Source: three-view drawing plus pictorial views. Frame: mm from the lowest corner of the part. Give positions to 0.01 mm unless a question says otherwise; leave off trailing zeros. Order: outer loops, then holes, each group sorted by start corner. A loop starts at its lowest first (then second) coordinate and runs counter-clockwise, first axis right, second up.
1) Section B-B, the plane x = 70. Return loops of the section in (y, z), plus the area to 3 significant figures.
2) Section A-A, the plane z = 50. Return loops of the section in (x, y) (1 decimal).
3) First-contact query: P1, Ø4, axis at x = 70, z = 89, coming from the -Y side; P2, Ø2, axis at x = 30, z = 89, coming from the +Y side; P3, Ø6, axis at x = 54, y = 3, coming from the -Z side; P4, Ø2, axis at x = 59, y = 10, coming from the +Z side. Flat tips, straight axial feed; report the tip coordinate or a pass-through.
4) Draft query along Y for the marked faces 1, 2 and 3. Return one class per face: released by +Y, released by -Y, zero draft, split by the parting line, or undercut.
5) Section D-D, the plane x = 54. Return loops of the section in (y, z).
6) Material intervals for line 1 (X direction, y = 15.6, z = 89); line 2 (X direction, y = 16.1, z = 15); line 3 (Y direction, x = 76, z = 84), sorted ascending.
7) Section C-C, the plane z = 15. Return loops of the section in (x, y).
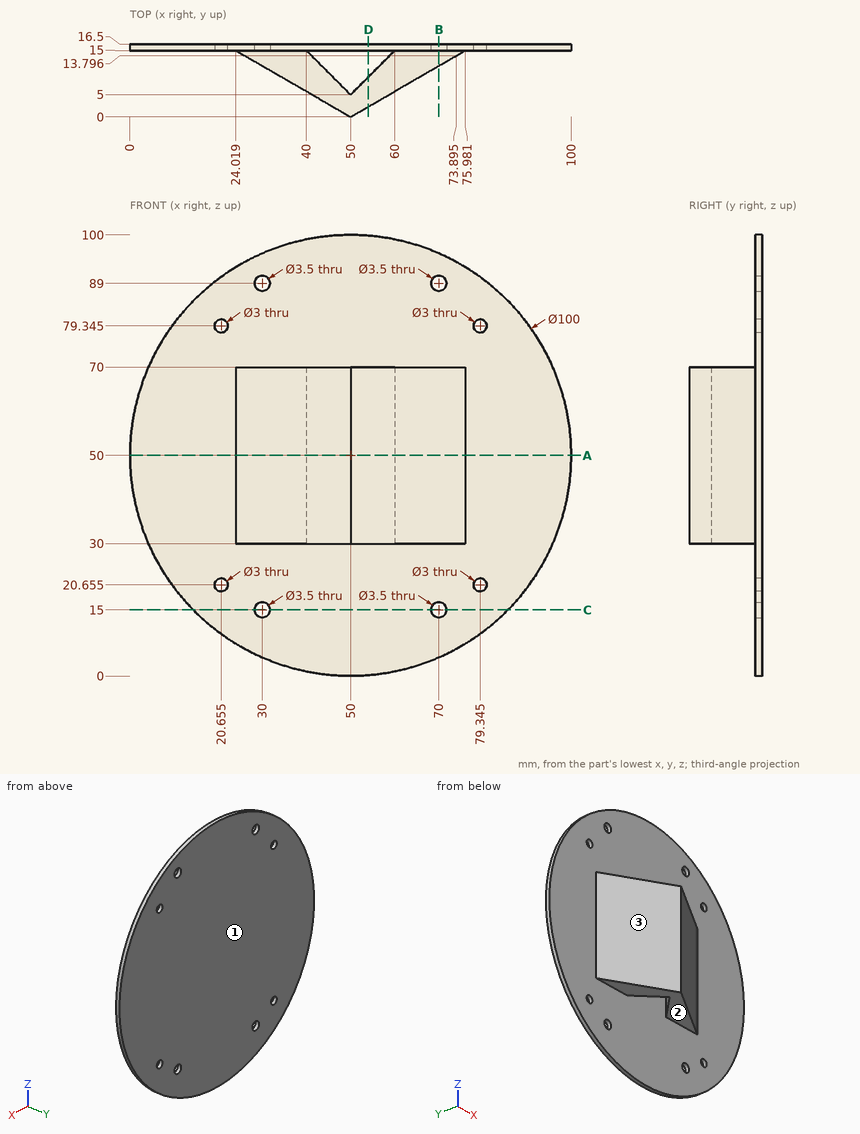
From the geometry:
1. outline: (11.55, 30) - (15, 30) - (15, 16.75) - (16.5, 16.75) - (16.5, 87.25) - (15, 87.25) - (15, 70) - (11.55, 70) - close; (15, 4.17) - (16.5, 4.17) - (16.5, 13.25) - (15, 13.25) - close; (15, 90.75) - (16.5, 90.75) - (16.5, 95.83) - (15, 95.83) - close
1. area: 265 mm2
2. outline: (0, 15) - (24, 15) - (50, 0) - (73.9, 13.8) - (76, 15) - (100, 15) - (100, 16.5) - (0, 16.5) - close; hole (40, 15) - (50, 5) - (60, 15) - close
3. P1: stops at y = 15
3. P2: passes through
3. P3: stops at z = 30
3. P4: stops at z = 70
4. face 1: released by +Y
4. face 2: zero draft
4. face 3: released by -Y
5. outline: (2.31, 30) - (9, 30) - (9, 70) - (2.31, 70) - close; (15, 0.16) - (16.5, 0.16) - (16.5, 99.84) - (15, 99.84) - close
6. line 1: x = 18.71 to 28.25, 31.75 to 68.25, 71.75 to 81.29
6. line 2: x = 14.29 to 28.25, 31.75 to 68.25, 71.75 to 85.71
6. line 3: y = 15 to 16.5
7. outline: (14.29, 15) - (28.25, 15) - (28.25, 16.5) - (14.29, 16.5) - close; (31.75, 15) - (68.25, 15) - (68.25, 16.5) - (31.75, 16.5) - close; (71.75, 15) - (85.71, 15) - (85.71, 16.5) - (71.75, 16.5) - close
